Input: part model. Units: mm. Frame: model coordinates. Coordinates: 2 decimals unless noted, no trailing zeros. Write each loop counter-clockwise with the first axis right and the second up, starting at its lowest first coordinate (ties: lowest second). Pieces come first, ordered by that corner, then holes. Notation, with made-up numbers: (30.5, 68) - (55.5, 68) arc R12 cw to (55.5, 79) - close; hole circle Ø11 at (-9.75, -3). An arc over 180 degrees is marked (long way). Put each result on its own line as item: value. Start each with the question number.
1. Cut plane C-C, the plane z = 0.85. Count the separate pieces of the cut face and the enclosed holes in it, and give its area (3 significant figures).
2. Cut plane D-D, the plane x = -36. Return loops of the section in (y, z).
3. Line query: line 1 (X direction, y = -22, z = 0.7); line 2 (X direction, y = -44, z = 0.35); line 3 (Y direction, x = -21, z = 0.2). Output: solid intervals per line, ascending.
4. Cut plane B-B, the plane y = 0. Return loops of the section in (x, z).
5. Cut plane A-A, the plane x = 0. Return loops of the section in (y, z), and give its area (3 significant figures).
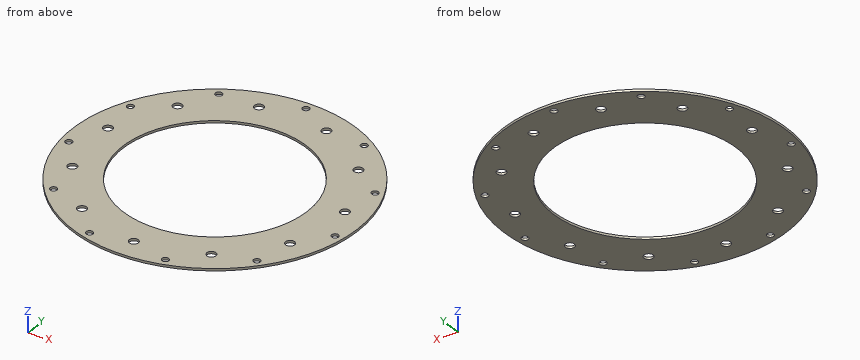
from build123d import *

# Parameters (mm, degrees)
SKETCH_1_R      = 62.5
SKETCH_1_R_2    = 40.5
SKETCH_1_R_3    = 2
SKETCH_1_R_4    = 1.5
EXTRUDE_1_DEPTH = 1


with BuildPart() as part:
    # 草图1 → 凸台-拉伸1 (new body)
    with BuildSketch(Plane.XY):
        Circle(SKETCH_1_R)
        Circle(SKETCH_1_R_2, mode=Mode.SUBTRACT)
        with Locations((0, -52.5)):
            Circle(SKETCH_1_R_3, mode=Mode.SUBTRACT)
        with Locations((-28.383642916, -44.165810474)):
            Circle(SKETCH_1_R_3, mode=Mode.SUBTRACT)
        with Locations((-47.755679756, -21.809288183)):
            Circle(SKETCH_1_R_3, mode=Mode.SUBTRACT)
        with Locations((-51.965625699, 7.471529009)):
            Circle(SKETCH_1_R_3, mode=Mode.SUBTRACT)
        with Locations((-39.676852654, 34.380188532)):
            Circle(SKETCH_1_R_3, mode=Mode.SUBTRACT)
        with Locations((-14.790959234, 50.373381115)):
            Circle(SKETCH_1_R_3, mode=Mode.SUBTRACT)
        with Locations((14.790959234, 50.373381115)):
            Circle(SKETCH_1_R_3, mode=Mode.SUBTRACT)
        with Locations((39.676852654, 34.380188532)):
            Circle(SKETCH_1_R_3, mode=Mode.SUBTRACT)
        with Locations((51.965625699, 7.471529009)):
            Circle(SKETCH_1_R_3, mode=Mode.SUBTRACT)
        with Locations((47.755679756, -21.809288183)):
            Circle(SKETCH_1_R_3, mode=Mode.SUBTRACT)
        with Locations((28.383642916, -44.165810474)):
            Circle(SKETCH_1_R_3, mode=Mode.SUBTRACT)
        with Locations((-16.622220854, -56.610085443)):
            Circle(SKETCH_1_R_4, mode=Mode.SUBTRACT)
        with Locations((-44.589224887, -38.636783303)):
            Circle(SKETCH_1_R_4, mode=Mode.SUBTRACT)
        with Locations((-58.399465071, -8.396575458)):
            Circle(SKETCH_1_R_4, mode=Mode.SUBTRACT)
        with Locations((-53.668287726, 24.509485767)):
            Circle(SKETCH_1_R_4, mode=Mode.SUBTRACT)
        with Locations((-31.89780823, 49.633958437)):
            Circle(SKETCH_1_R_4, mode=Mode.SUBTRACT)
        with Locations((0, 59)):
            Circle(SKETCH_1_R_4, mode=Mode.SUBTRACT)
        with Locations((31.89780823, 49.633958437)):
            Circle(SKETCH_1_R_4, mode=Mode.SUBTRACT)
        with Locations((53.668287726, 24.509485767)):
            Circle(SKETCH_1_R_4, mode=Mode.SUBTRACT)
        with Locations((58.399465071, -8.396575458)):
            Circle(SKETCH_1_R_4, mode=Mode.SUBTRACT)
        with Locations((44.589224887, -38.636783303)):
            Circle(SKETCH_1_R_4, mode=Mode.SUBTRACT)
        with Locations((16.622220854, -56.610085443)):
            Circle(SKETCH_1_R_4, mode=Mode.SUBTRACT)
    extrude(amount=EXTRUDE_1_DEPTH)


solid = part.part
Report:
1. separate pieces: 1
1. enclosed holes: 23
1. area: 6,900 mm^2
2. outline: (-51.09, 0) - (-18.55, 0) - (-18.55, 1) - (-51.09, 1) - close; (18.55, 0) - (51.09, 0) - (51.09, 1) - (18.55, 1) - close
3. line 1: x = -58.5 to -49.75, -45.76 to -34, 34 to 45.76, 49.75 to 58.5
3. line 2: x = -44.39 to -30.38, -26.39 to 26.39, 30.38 to 44.39
3. line 3: y = -58.87 to -34.63, 34.63 to 58.87
4. outline: (-62.5, 0) - (-40.5, 0) - (-40.5, 1) - (-62.5, 1) - close; (40.5, 0) - (62.5, 0) - (62.5, 1) - (40.5, 1) - close
5. outline: (-62.5, 0) - (-54.5, 0) - (-54.5, 1) - (-62.5, 1) - close; (-50.5, 0) - (-40.5, 0) - (-40.5, 1) - (-50.5, 1) - close; (40.5, 0) - (57.5, 0) - (57.5, 1) - (40.5, 1) - close; (60.5, 0) - (62.5, 0) - (62.5, 1) - (60.5, 1) - close
5. area: 37.0 mm^2
